Source: CAD feature listing. Evaluate the final solid. Frame: model axes, mm. A direction names the side the tool comes from. Coordinates: 2 decimals unless noted, no trailing zeros. Order: outer loops, then holes, each group sorted by start corner. A loop starts at its lowest first (then second) coordinate and runs counter-clockwise, first axis right, second up. Notation, with made-up numbers: (17, 51.5) -> (30, 51.5) arc R23 ccw to (30, 67.5) -> close; hole circle Ø10 at (-32, -1). An arc over 180 degrees is marked (long way). Write item = value, one per line. Start each with the question number.
Item 1: Ray query, line 1 along Y through (x, z) = (0, 4.5); line 2 along Y through (x, z) = (1, 3); line 3 along X through (y, z) = (50.5, 6). Return the intervals inside material, ascending. Write a range as [from, to].
Item 2: Section query B-B (y = 11.5). Output: boundary loops of the cut face in (x, z) (1 decimal), then the cut area to 3 significant figures.
Item 3: Mould query, pull axis X, two halves, no side actions, for faces 1 (the cylindrical face through (3.37, 28.17, 5.88)), 2 (the cylindrical face through (-0.3, 9.25, 3.47)), 3 (the flat face through (-2.7, 28.2, 6.839)). Classes: released by +X, released by -X, zero draft, split by the parting line, or undercut.
Item 4: Set-up query: faces 4 (the flat face through (-5.321, 28.175, 2.495)), 5 (the flat face through (5, 28, 5.474)), 6 (the flat face through (-5, 28, 5.474)). Return all of +Z, -Z, +X, -X, +Y, -Y with unobstructed straight access to the full face (end or side cutting, diameter ignored); none if empty.
Item 5: Section query A-A (x = 0). Output: boundary loops of the cut face in (y, z).
Item 6: Contact query for flat-ended pins moving along their axis: pin 1 (4 mm diameter, centred on x = 0, y = 50.165, fed in from +Z); pin 2 (2.5 mm diameter, centred on x = -5.5, y = 31, fed in from +Z); pin 3 (3 mm diameter, centred on x = 4, y = 46.5, fed in from +Z); pin 4 (2.5 mm diameter, centred on x = 5, y = 21.5, fed in from +Z). Output: stop coordinate, or through.
Item 7: Section query C-C (z = 2.75). Output: boundary loops of the cut face in (x, y) (3 decimals), then the cut area to 3 significant figures.
```python
from build123d import *

# Parameters (mm, degrees)
BOSS_EXTRUDE1_DEPTH = 57.15
SKETCH2_R           = 2.286
CUT_EXTRUDE1_DEPTH  = 7.8393


with BuildPart() as part:
    # Sketch1 → Boss-Extrude1 (new body)
    with BuildSketch(Plane(origin=(0, 0, 0), x_dir=(1, 0, 0), z_dir=(0, 1, 0))):
        with BuildLine():
            Line((-2.9785, -6.8393), (2.978499971, -6.8393))
            ThreePointArc((2.978499971, -6.8393), (3.378269925, -5.874169954), (4.343399971, -5.4744))
            Line((4.343399971, -5.4744), (6.474794456, -5.4744))
            ThreePointArc((6.474794456, -5.4744), (7.173247382, -5.007708675), (7.009367182, -4.183827273))
            Line((7.009367182, -4.183827273), (3.679323642, -0.853783733))
            ThreePointArc((3.679323642, -0.853783733), (2.73362958, -0.221891163), (1.618107374, 0))
            Line((1.618107374, 0), (-1.618107374, 0))
            ThreePointArc((-1.618107374, 0), (-2.73362958, -0.221891163), (-3.679323642, -0.853783733))
            Line((-3.679323642, -0.853783733), (-7.009367182, -4.183827273))
            ThreePointArc((-7.009367182, -4.183827273), (-7.173247382, -5.007708675), (-6.474794456, -5.4744))
            Line((-6.474794456, -5.4744), (-4.3434, -5.4744))
            ThreePointArc((-4.3434, -5.4744), (-3.378269954, -5.874169954), (-2.9785, -6.8393))
        make_face()
    extrude(amount=BOSS_EXTRUDE1_DEPTH)

    # Sketch2 → Cut-Extrude1 (cut, through all)
    with BuildSketch(Plane.XY.offset(6.8393)):
        with Locations((0, 50.165)):
            Circle(SKETCH2_R)
        with Locations((0, 28.575)):
            Circle(SKETCH2_R)
        with Locations((0, 6.985)):
            Circle(SKETCH2_R)
    extrude(amount=-CUT_EXTRUDE1_DEPTH, mode=Mode.SUBTRACT)


solid = part.part
```
Computed:
q1.line_1 = [0, 4.7], [9.27, 26.29], [30.86, 47.88], [52.45, 57.15]
q1.line_2 = [0, 4.93], [9.04, 26.52], [30.63, 48.11], [52.22, 57.15]
q1.line_3 = [-3.27, -2.26], [2.26, 3.27]
q2.outline = (-7, 4.2) -> (-3.7, 0.9) arc R2.9 ccw to (-1.6, 0) -> (1.6, 0) arc R2.9 ccw to (3.7, 0.9) -> (7, 4.2) arc R0.8 ccw to (6.5, 5.5) -> (4.3, 5.5) arc R1.4 cw to (3, 6.8) -> (-3, 6.8) arc R1.4 cw to (-4.3, 5.5) -> (-6.5, 5.5) arc R0.8 ccw to start
q2.area = 68.1 mm^2
q3.face_1 = released by +X
q3.face_2 = undercut
q3.face_3 = zero draft
q4.face_4 = -Z, -X, +Y, -Y
q4.face_5 = +Z, +X, +Y, -Y
q4.face_6 = +Z, -X, +Y, -Y
q5.outline = (0, 0) -> (4.7, 0) -> (4.7, 6.84) -> (0, 6.84) -> close; (9.27, 0) -> (26.29, 0) -> (26.29, 6.84) -> (9.27, 6.84) -> close; (30.86, 0) -> (47.88, 0) -> (47.88, 6.84) -> (30.86, 6.84) -> close; (52.45, 0) -> (57.15, 0) -> (57.15, 6.84) -> (52.45, 6.84) -> close
q6.pin_1 = through
q6.pin_2 = 5.48
q6.pin_3 = 6.84
q6.pin_4 = 5.61
q7.outline = (-5.576, 0) -> (5.576, 0) -> (5.576, 57.15) -> (-5.576, 57.15) -> close; hole circle Ø4.572 at (0, 6.985); hole circle Ø4.572 at (0, 28.575); hole circle Ø4.572 at (0, 50.165)
q7.area = 588 mm^2
